Geometry check sheet. Reference: drawing and pictorial views, mm from the part's lowest x, y, z. A direction names the side the tool comes from. Give positions to 0.01 mm unless a question says otherwise; leave off trailing zeros. Order: outer loops, then holes, each group sorted by start corner. A loop starts at its lowest first (then second) coordinate and runs counter-clockwise, first axis right, second up.
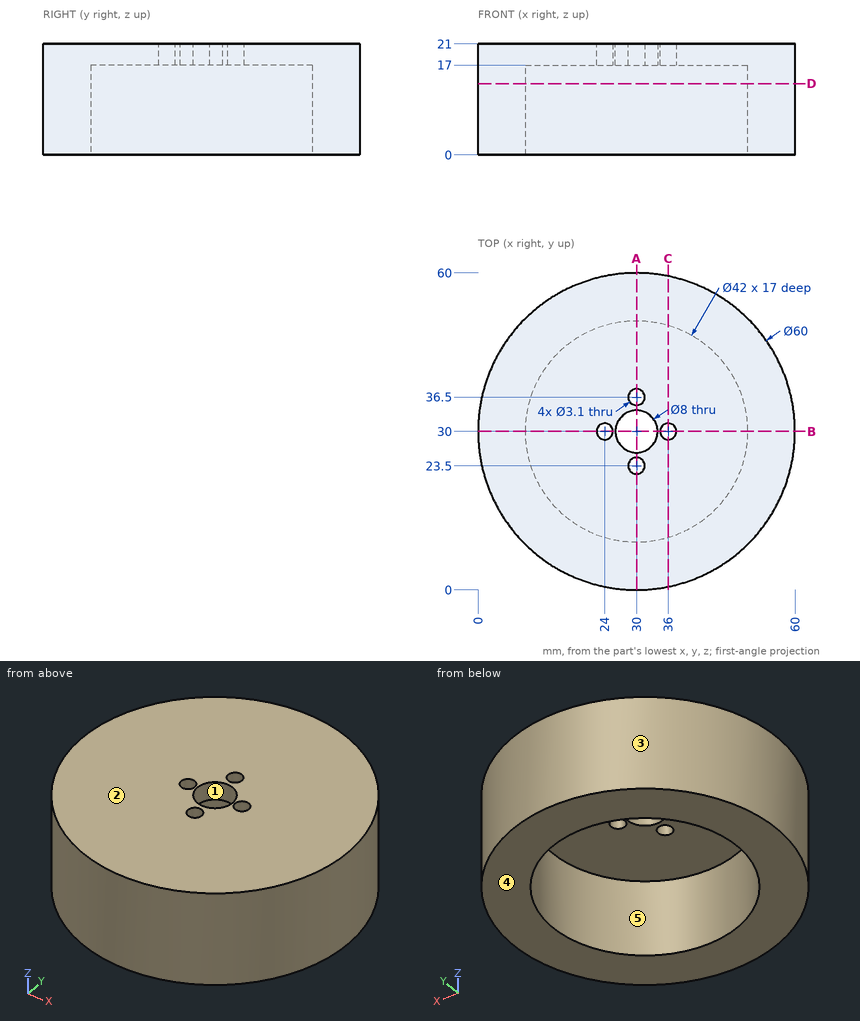
1) Depth check by flat-ended pin: pin 1 Ø3.5 at (x, y) = (24, 30) entering from -Z; pin 2 Ø4 at (y, z) = (13, 19) entering from +X; pin 3 Ø1 at (y, z) = (47, 12.5) entering from -X; pin 4 Ø4 at (x, y) = (30, 23.5) entering from +Z. Enter the tip coordinate at first touch or a pass-through.
Recorded:
pin 1: stops at z = 17
pin 2: stops at x = 55.98
pin 3: stops at x = 4.95
pin 4: stops at z = 21
2) Section check B-B, the plane y = 30. Record the cut outline in (x, z), then the cut area to 3 significant figures.
Recorded:
outline: (0, 0) - (9, 0) - (9, 17) - (22.45, 17) - (22.45, 21) - (0, 21) - close; (25.55, 17) - (26, 17) - (26, 21) - (25.55, 21) - close; (34, 17) - (34.45, 17) - (34.45, 21) - (34, 21) - close; (37.55, 17) - (51, 17) - (51, 0) - (60, 0) - (60, 21) - (37.55, 21) - close
area: 489 mm2
3) Section check D-D, the plane z = 13.5. Record the cut outline in (x, y).
Recorded:
outline: circle Ø60 at (30, 30); hole circle Ø42 at (30, 30)
4) Section check A-A, the plane x = 30. Record the cut outline in (y, z).
Recorded:
outline: (0, 0) - (9, 0) - (9, 17) - (21.95, 17) - (21.95, 21) - (0, 21) - close; (25.05, 17) - (26, 17) - (26, 21) - (25.05, 21) - close; (34, 17) - (34.95, 17) - (34.95, 21) - (34, 21) - close; (38.05, 17) - (51, 17) - (51, 0) - (60, 0) - (60, 21) - (38.05, 21) - close
5) Draft check along Y on the marked faces 1, 2 and 3. Enter one of: +Y half, -Y half, draft (parallel to the pull), parting line (faces both ways), or undercut.
Recorded:
face 1: undercut
face 2: draft
face 3: parting line
6) Set-up check for the marked faces 4 and 5: record each of +Z, -Z, +X, -X, +Y, -Y from which the full face is reachable in a straight line by a thin tool's end or side.
Recorded:
face 4: -Z, +X, -X, +Y, -Y
face 5: -Z
7) Section check C-C, the plane x = 36. Record the cut outline in (y, z).
Recorded:
outline: (0.61, 0) - (9.88, 0) - (9.88, 17) - (28.45, 17) - (28.45, 21) - (0.61, 21) - close; (31.55, 17) - (50.12, 17) - (50.12, 0) - (59.39, 0) - (59.39, 21) - (31.55, 21) - close
8) Material ranges on L1, parallel to Y at x = 30, z = 19.4; L2, parallel to Y at x = 29.5, z = 16; L3, parallel to Z at x = 22.5, y = 28.5, recorded low to high.
Recorded:
L1: y = 0 to 21.95, 25.05 to 26, 34 to 34.95, 38.05 to 60
L2: y = 0 to 9.01, 50.99 to 60
L3: z = 17 to 21
